Part model, mm, in its own coordinate system. A direction names the side the tool comes from. Round coordinates to 2 decimals unless told otherwise and drop trailing zeros. Loops run counter-clockwise (first coordinate to the right, second up) from the corner with the lowest first, then second, coordinate; pieces in that order, holes last. Notation, with made-up numbers: (-12, -34) -> (3, -34) arc R15 ccw to (3, -25) -> close; hole circle Ø6 at (34, -34.75). An arc over 180 degrees is marked (long way). Use a Markdown table: item, result. Add a question column.
Item 1: Flat gauge pins, fed straight in: pin 1 (1.5 mm diameter, centred on y = 37, z = 2, fed in from -X); pin 2 (2.5 mm diameter, centred on x = 65, y = 0, fed in from +Z); pin 3 (1 mm diameter, centred on x = -46, z = 0.5, fed in from +Y); pin 4 (1.5 mm diameter, centred on y = 41, z = 1.5, fed in from +X). Where does each tip first touch, or does it go through?
Item 2: Two-plate mould, pull along X, no slides. Class faces 1 (the face through (-20, 43, 1)), 2 (the face through (66.43, 0.45, 1.27)), 3 (the face through (11.733, 63.932, 1.479)): pulls with the +X half, pulls with the -X half, needs draft (parallel to the pull), parting line crosses it, or undercut.
Item 3: Which spindle directions (+Z, -Z, +X, -X, +Y, -Y) get a long thin tool onto all of the face, cutting with end or side? Do faces 4 (the face through (-42, 25, 1)), 5 (the face through (-20, -44, 1)), 6 (the face through (40, 25, 1)). Say none if no direction does.
Item 4: Cut at A-A, the plane z = 1.05. List the corners of the cut face in (x, y).
Item 5: Cut at C-C, the plane y = -45. List the corners of the cut face in (x, z).
Item 6: Probe line 1 (Y direction, x = 0, z = 0.85); line 2 (Y direction, x = 65, z = 1.05); line 3 (Y direction, x = 38, z = 0.4). List the from-to ranges inside material, lowest first. Write a range as [from, to].
Item 7: Cut at B-B, the plane x = 49. List the corners of the cut face in (y, z), plus the area to 3 significant figures.
```python
from build123d import *

# Parameters (mm, degrees)
EXTRUDE_1_DEPTH     = 3
SKETCH_2_R          = 3.5
EXTRUDE_2_DEPTH     = 3
SKETCH_3_R          = 1.5
CUT_EXTRUDE_1_DEPTH = 3
CHAMFER_1_SIZE      = 0.5
EXTRUDE_START       = -3
EXTRUDE_4_DEPTH     = 3


with BuildPart() as part:
    # 草图1 → 凸台-拉伸1 (new body)
    with BuildSketch(Plane.XY):
        with BuildLine():
            Line((20, -25), (20, -61.846584384))
            ThreePointArc((20, -61.846584384), (0, -65), (-20, -61.846584384))
            Line((-20, -61.846584384), (-20, -25))
            Line((-20, -25), (-60, -25))
            ThreePointArc((-60, -25), (-65, 0), (-60, 25))
            Line((-60, 25), (-20, 25))
            Line((-20, 25), (-20, 61.846584384))
            ThreePointArc((-20, 61.846584384), (0, 65), (20, 61.846584384))
            Line((20, 61.846584384), (20, 25))
            Line((20, 25), (60, 25))
            ThreePointArc((60, 25), (65, 0), (60, -25))
            Line((60, -25), (20, -25))
        make_face()
    extrude(amount=EXTRUDE_1_DEPTH)

    # 草图2 → 凸台-拉伸2 (add)
    with BuildSketch(Plane.XY.offset(3)):
        with Locations((65, 0)):
            Circle(SKETCH_2_R)
        with Locations((0, 65)):
            Circle(SKETCH_2_R)
        with Locations((0, -65)):
            Circle(SKETCH_2_R)
    extrude(amount=-EXTRUDE_2_DEPTH)

    # 草图3 → 切除-拉伸1 (cut)
    with BuildSketch(Plane.XY.offset(3)):
        with Locations((0, 65)):
            Circle(SKETCH_3_R)
        with Locations((65, 0)):
            Circle(SKETCH_3_R)
        with Locations((0, -65)):
            Circle(SKETCH_3_R)
    extrude(amount=-CUT_EXTRUDE_1_DEPTH, mode=Mode.SUBTRACT)

    # 倒角1
    chamfer_1_edges = [part.edges().sort_by_distance(p)[0] for p in [
        (-1.5, 65, 3),
        (63.5, 0, 3),
        (-1.5, -65, 3),
    ]]
    chamfer(chamfer_1_edges, length=CHAMFER_1_SIZE)

    # 草图4 → 凸台-拉伸4 (add)
    with BuildSketch(Plane.XY.offset(3).offset(EXTRUDE_START)):
        with BuildLine():
            ThreePointArc((-60, -25), (-63.73774392, -12.747548784), (-65, 0))
            Line((-65, 0), (-65, -25))
            Line((-65, -25), (-60, -25))
        make_face()
        with BuildLine():
            ThreePointArc((-65, 0), (-63.73774392, 12.747548784), (-60, 25))
            Line((-60, 25), (-65, 25))
            Line((-65, 25), (-65, 0))
        make_face()
    extrude(amount=EXTRUDE_4_DEPTH)


solid = part.part
```
A:
| question | item | result |
|---|---|---|
| 1 | pin 1 | stops at x = -20 |
| 1 | pin 2 | passes through |
| 1 | pin 3 | stops at y = 25 |
| 1 | pin 4 | stops at x = 20 |
| 2 | face 1 | pulls with the -X half |
| 2 | face 2 | undercut |
| 2 | face 3 | pulls with the +X half |
| 3 | face 4 | +Z, -Z, -X, +Y |
| 3 | face 5 | +Z, -Z, -X, -Y |
| 3 | face 6 | +Z, -Z, +X, +Y |
| 4 | outline | (-65, -25) -> (-20, -25) -> (-20, -61.85) arc R65 ccw to (-3.5, -64.91) arc R3.5 ccw (long way) to (3.5, -64.91) arc R65 ccw to (20, -61.85) -> (20, -25) -> (60, -25) arc R65 ccw to (64.91, -3.5) arc R3.5 ccw (long way) to (64.91, 3.5) arc R65 ccw to (60, 25) -> (20, 25) -> (20, 61.85) arc R65 ccw to (3.5, 64.91) arc R3.5 ccw (long way) to (-3.5, 64.91) arc R65 ccw to (-20, 61.85) -> (-20, 25) -> (-65, 25) -> close; hole circle Ø3 at (0, -65); hole circle Ø3 at (0, 65); hole circle Ø3 at (65, 0) |
| 5 | outline | (-20, 0) -> (20, 0) -> (20, 3) -> (-20, 3) -> close |
| 6 | line 1 | y = [-68.5, -66.5], [-63.5, 63.5], [66.5, 68.5] |
| 6 | line 2 | y = [-3.5, -1.5], [1.5, 3.5] |
| 6 | line 3 | y = [-25, 25] |
| 7 | outline | (-25, 0) -> (25, 0) -> (25, 3) -> (-25, 3) -> close |
| 7 | area | 150 mm^2 |
